CAD build for the part. Positions are in the model's coordinates, mm. Face numbers are marked on the shaded views. A direction names the side the tool comes from. Coordinates: 2 decimals unless noted, no trailing zeros. Loops run counter-clockwise (first coordinate to the right, second up) from the corner with the lowest first, then second, coordinate; pieces in that order, holes last.
1) Saw through at C-C, the plane z = 9. Write the cut outline in (x, y).
2) Pin check, flat tips, straight feed: pin 1 Ø4 at (x, y) = (-10, -20) entering from -Z; pin 2 Ø0.8 at (x, z) = (-3.5, 34) entering from +Y; pin 3 Ø7 at (x, y) = (9.5, 18) entering from +Z; pin 4 Ø8 at (y, z) = (0, 32.5) entering from +X. Stop position of each tip, or through.
3) Saw through at A-A, the plane y = -20. Write the cut outline in (x, z), and give its area (3 significant figures).
4) Saw through at D-D, the plane z = 37. Write the cut outline in (x, y), and give its area (4 significant figures).
5) Wall check: line 1 along Y through (x, z) = (10, 2); line 2 along Y through (x, z) = (10, 8); line 3 along Z through (x, y) = (-13.5, 12). Give the ranges that are in metal, low to high.
6) Which spindle directions (+Z, -Z, +X, -X, +Y, -Y) get a long thin tool onto all of the face, cutting with end or side? Do the marked faces 1, 2 and 3. Say none if no direction does.
7) Saw through at B-B, the plane x = 10. Write the cut outline in (y, z), and give its area (3 significant figures).
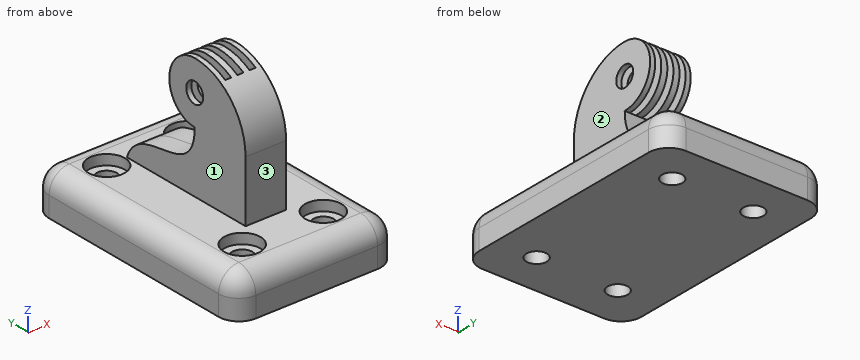
```python
from build123d import *

# Parameters (mm, degrees)
SKETCH1_W           = 40
SKETCH1_H           = 60
BOSS_EXTRUDE1_DEPTH = 10
SKETCH2_R           = 2.5
CUT_EXTRUDE1_DEPTH  = 10
FILLET1_R           = 5
FILLET2_R           = 5
BOSS_EXTRUDE2_DEPTH = 5
CUT_EXTRUDE2_DEPTH  = 0.75
LPATTERN1_COUNT     = 2
LPATTERN1_PITCH     = 3
LPATTERN2_COUNT     = 2
LPATTERN2_PITCH     = 3
SKETCH5_R           = 4.5
CUT_EXTRUDE3_DEPTH  = 2.5
SKETCH6_R           = 2.5
CUT_EXTRUDE4_DEPTH  = 23.5


with BuildPart() as part:
    # Sketch1 → Boss-Extrude1 (new body)
    with BuildSketch(Plane.XY):
        Rectangle(SKETCH1_W, SKETCH1_H)
    extrude(amount=BOSS_EXTRUDE1_DEPTH)

    # Sketch2 → Cut-Extrude1 (cut)
    with BuildSketch(Plane.XY.offset(10)):
        with Locations((-10, -20)):
            Circle(SKETCH2_R)
        with Locations(Location((10, -20, 0), (0, 0, 180))):
            Circle(SKETCH2_R)
        with Locations((10, 20)):
            Circle(SKETCH2_R)
        with Locations(Location((-10, 20, 0), (0, 0, 180))):
            Circle(SKETCH2_R)
    extrude(amount=-CUT_EXTRUDE1_DEPTH, mode=Mode.SUBTRACT)

    # Fillet1
    fillet1_edges = [part.edges().sort_by_distance(p)[0] for p in [
        (20, -30, 5),
        (-20, -30, 5),
        (-20, 30, 5),
        (20, 30, 5),
    ]]
    fillet(fillet1_edges, radius=FILLET1_R)

    # Fillet2
    fillet2_edges = [part.edges().sort_by_distance(p)[0] for p in [
        (0, 30, 10),
        (20, 0, 10),
        (-20, 0, 10),
        (0, -30, 10),
        (-18.535533906, 28.535533906, 10),
        (-18.535533906, -28.535533906, 10),
        (18.535533906, -28.535533906, 10),
        (18.535533906, 28.535533906, 10),
    ]]
    fillet(fillet2_edges, radius=FILLET2_R)

    # Sketch3 → Boss-Extrude2 (add, symmetric)
    with BuildSketch(Plane(origin=(0, 0, 0), x_dir=(0, 0, -1), z_dir=(1, 0, 0))):
        with BuildLine():
            Line((-10, -15), (-25, -15))
            ThreePointArc((-25, -15), (-35.606601718, -10.606601718), (-40, 0))
            ThreePointArc((-40, 0), (-32.5, 7.5), (-25, 0))
            add(Edge.make_bspline(
                [(-25, 0), (-11.206458261, 0.023360815), (-20.592449016, 16.330430805), (-10, 20)],
                knots=[0, 0, 0, 0, 1, 1, 1, 1], degree=3))
            Line((-10, 20), (-10, -15))
        make_face()
    extrude(amount=BOSS_EXTRUDE2_DEPTH, both=True)

    # Sketch4 → Cut-Extrude2 (cut, symmetric)
    with BuildSketch(Plane(origin=(0, 0, 0), x_dir=(0, 0, -1), z_dir=(1, 0, 0))):
        with BuildLine():
            Line((-32.5, -7.5), (-40, -7.5))
            Line((-40, -7.5), (-40, 0))
            ThreePointArc((-40, 0), (-27.196699141, 5.303300859), (-32.5, -7.5))
        make_face()
    cut_extrude2 = extrude(amount=CUT_EXTRUDE2_DEPTH, both=True, mode=Mode.SUBTRACT)

    # LPattern1: Cut-Extrude2 ×2
    with Locations(*[(-i * LPATTERN1_PITCH, 0, 0) for i in range(1, LPATTERN1_COUNT)]):
        add(cut_extrude2, mode=Mode.SUBTRACT)

    # LPattern2: Cut-Extrude2 ×2
    with Locations(*[(i * LPATTERN2_PITCH, 0, 0) for i in range(1, LPATTERN2_COUNT)]):
        add(cut_extrude2, mode=Mode.SUBTRACT)

    # Sketch5 → Cut-Extrude3 (cut, symmetric)
    with BuildSketch(Plane.XY.offset(10)):
        with Locations(Location((-10, -20, 0), (0, 0, 180))):
            Circle(SKETCH5_R)
        with Locations((-10, 20)):
            Circle(SKETCH5_R)
        with Locations((10, -20)):
            Circle(SKETCH5_R)
        with Locations(Location((10, 20, 0), (0, 0, 180))):
            Circle(SKETCH5_R)
    extrude(amount=CUT_EXTRUDE3_DEPTH, both=True, mode=Mode.SUBTRACT)

    # Sketch6 → Cut-Extrude4 (cut, symmetric)
    with BuildSketch(Plane(origin=(5, 0, 0), x_dir=(0, 0, -1), z_dir=(1, 0, 0))):
        with Locations((-32.5, 0)):
            Circle(SKETCH6_R)
    extrude(amount=CUT_EXTRUDE4_DEPTH, both=True, mode=Mode.SUBTRACT)


solid = part.part
```
Data:
1. outline: (-18, -25) arc R3 ccw to (-15, -28) - (15, -28) arc R3 ccw to (18, -25) - (18, 25) arc R3 ccw to (15, 28) - (-15, 28) arc R3 ccw to (-18, 25) - close; hole circle Ø9 at (-10, -20); hole circle Ø9 at (-10, 20); hole circle Ø9 at (10, -20); hole circle Ø9 at (10, 20)
2. pin 1: passes through
2. pin 2: stops at y = 7.41
2. pin 3: stops at z = 10
2. pin 4: stops at x = 5
3. outline: (-20, 0) - (-12.5, 0) - (-12.5, 7.5) - (-14.5, 7.5) - (-14.5, 10) - (-15, 10) arc R5 ccw to (-20, 5) - close; (-7.5, 0) - (7.5, 0) - (7.5, 7.5) - (5.5, 7.5) - (5.5, 10) - (-5.5, 10) - (-5.5, 7.5) - (-7.5, 7.5) - close; (12.5, 0) - (20, 0) - (20, 5) arc R5 ccw to (15, 10) - (14.5, 10) - (14.5, 7.5) - (12.5, 7.5) - close
3. area: 269 mm2
4. outline: (-5, -9) - (5, -9) - (5, 6) - (3.75, 6) - (3.75, -7.5) - (2.25, -7.5) - (2.25, 6) - (0.75, 6) - (0.75, -7.5) - (-0.75, -7.5) - (-0.75, 6) - (-2.25, 6) - (-2.25, -7.5) - (-3.75, -7.5) - (-3.75, 6) - (-5, 6) - close
4. area: 89.25 mm2
5. line 1: y = -30 to -22.5, -17.5 to 17.5, 22.5 to 30
5. line 2: y = -29 to -24.5, -15.5 to 15.5, 24.5 to 29
5. line 3: z = 0 to 10
6. face 1: +Z, -X, +Y, -Y
6. face 2: +Z, +X, +Y, -Y
6. face 3: +Z, +X, -X, -Y
7. outline: (-30, 0) - (-22.5, 0) - (-22.5, 7.5) - (-24.5, 7.5) - (-24.5, 10) - (-25, 10) arc R5 ccw to (-30, 5) - close; (-17.5, 0) - (17.5, 0) - (17.5, 7.5) - (15.5, 7.5) - (15.5, 10) - (-15.5, 10) - (-15.5, 7.5) - (-17.5, 7.5) - close; (22.5, 0) - (30, 0) - (30, 5) arc R5 ccw to (25, 10) - (24.5, 10) - (24.5, 7.5) - (22.5, 7.5) - close
7. area: 469 mm2
